Input: part model. Units: mm. Frame: model coordinates. A direction names the side the tool comes from. Give positions to 0.01 mm unless a question says otherwise; leave off trailing zeros. Loops run counter-clockwise (first coordinate to the right, second up) from the corner with the lowest first, then second, coordinate; pieces in that order, holes last.
from build123d import *

# Parameters (mm, degrees)
F2_R     = 1.9812
F3_DEPTH = 11.1262
F4_T     = -2.3876


with BuildPart() as f1:
    # F0 (on Front) → F1 (revolve)
    with BuildSketch(Plane.XZ):
        with BuildLine():
            Line((-2.756924, 12.7), (-5.5626, 12.7))
            Line((-5.5626, 12.7), (-5.5626, 0))
            Line((-5.5626, 0), (5.5626, 0))
            Line((5.5626, 0), (5.5626, 12.7))
            Line((5.5626, 12.7), (2.756924, 12.7))
            ThreePointArc((2.756924, 12.7), (0, 11.0998), (-2.756924, 12.7))
        make_face()
    revolve(axis=Axis((0, 0, 0), (1, 0, 0)))

    # F2 (on face) → F3 (cut, through all)
    with BuildSketch(Plane.YZ.offset(5.5626)):
        Circle(F2_R)
    extrude(amount=-F3_DEPTH, mode=Mode.SUBTRACT)

    # F4
    f4_openings = [f1.faces().sort_by_distance(p)[0] for p in [
        (-5.5626, 0, -12.34079),
    ]]
    offset(amount=F4_T, openings=f4_openings)


solid = f1.part
(1) Cut plane C-C (x = 5.25). Return the cut outline in (y, z).
Values follow:
outline: circle Ø25.4 at (0, 0); hole circle Ø3.96 at (0, 0)
(2) Mould query, pull axis Z, two halves, no side actions, for faces 4 (the flat face through (5.563, 0, -3)), 5 (the cylindrical face through (0.078, -0.258, 1.964)), 6 (the cylindrical face through (-4.18, 12.4, -2.75)). Classes: +Z half, -Z half, draft (parallel to the pull), parting line (faces both ways), or undercut.
Values follow:
face 4: draft
face 5: undercut
face 6: parting line
(3) Cut plane A-A (y = 0). Return the cut outline in (x, z) (3 decimals).
Values follow:
outline: (-5.563, -12.7) - (-2.757, -12.7) arc R3.175 cw to (2.757, -12.7) - (5.563, -12.7) - (5.563, -1.981) - (-5.563, -1.981) - (-5.563, -4.369) - (3.175, -4.369) - (3.175, -9.707) arc R5.563 ccw to (-3.904, -10.312) - (-5.563, -10.312) - close; (-5.563, 1.981) - (5.563, 1.981) - (5.563, 12.7) - (2.757, 12.7) arc R3.175 cw to (-2.757, 12.7) - (-5.563, 12.7) - (-5.563, 10.312) - (-3.904, 10.312) arc R5.563 ccw to (3.175, 9.707) - (3.175, 4.369) - (-5.563, 4.369) - close
(4) Reachability of faces 1 (the cylindrical face through (4.14, 12.4, -2.75)), 2 (the cylindrical face through (-1.133, 4.167, 1.312)), 3 (the flat face through (3.175, 4.2, -2)) from +Z, -Z, +X, -X, +Y, -Y: full face, straight path, thin tool, end or side. Return the list, or none.
Values follow:
face 1: +X, -X
face 2: -X
face 3: none
(5) Cut plane D-D (x = 0). Return the cut outline in (y, z).
Values follow:
outline: circle Ø22.2 at (0, 0); circle Ø8.74 at (0, 0); hole circle Ø17.42 at (0, 0); hole circle Ø3.96 at (0, 0)
(6) Pin query (flat end, axial travel): pin 1 Ø3 at (x, z) = (-1.5, -5.5) entering from -Y; pin 2 Ø5 at (x, z) = (2, -4.5) entering from -Y; pin 3 Ø2 at (x, z) = (-3, 9) entering from -Y. Return the tip coordinate at first contact, or that it passes through.
Values follow:
pin 1: stops at y = -11.81
pin 2: stops at y = -12.52
pin 3: stops at y = -9.86
(7) Ray query, probe 1 along Z at (x, y) = (-4.9, 0); probe 2 along Z at (x, y) = (0.75, 0.5); probe 3 along X at (y, z) = (-4.25, 2.25) (3 decimals). Return the intervals inside material, ascending.
Values follow:
probe 1: z = -12.7 to -10.31, -4.37 to -1.98, 1.98 to 4.37, 10.31 to 12.7
probe 2: z = -11.18 to -8.75, -4.34 to -1.92, 1.92 to 4.34, 8.75 to 11.18
probe 3: x = 3.175 to 5.563
